```python
from build123d import *

# Parameters (mm, degrees)
SKETCH_1_R      = 2.75
EXTRUDE_1_DEPTH = 10


with BuildPart() as part:
    # Эскиз1 → Бобышка-Вытянуть1 (new body)
    # profile 1 of 2: a face of its own
    with BuildSketch(Plane.XY):
        Polygon((-16, 0), (0, 0), (0, 14), (-2, 14), (-2, 15.226497308), (-12, 21), (-16, 21), align=None)
        with Locations((-9, 8)):
            Circle(SKETCH_1_R, mode=Mode.SUBTRACT)
    # profile 2 of 2: a face of its own
    with BuildSketch(Plane.XY):
        Polygon((0, 14), (0, 0), (16, 0), (16, 21), (12, 21), (2, 15.226497308), (2, 14), align=None)
        with Locations((9, 8)):
            Circle(SKETCH_1_R, mode=Mode.SUBTRACT)
    extrude(amount=EXTRUDE_1_DEPTH)


solid = part.part
```
Verification items for the finished model (mm, model axes). A direction names the side the tool comes from. Give positions to 0.01 mm unless a question says otherwise; leave off trailing zeros. Loops run counter-clockwise (first coordinate to the right, second up) from the corner with the lowest first, then second, coordinate; pieces in that order, holes last.
1. Section check D-D, the plane y = 16. Enter the section's corners in (x, z), then the cut area to 3 significant figures.
2. Set-up check for faces 1 (the flat face through (-2, 15, 5)), 2 (the flat face through (-14, 21, 5)): record each of +Z, -Z, +X, -X, +Y, -Y from which the full face is reachable in a straight line by a thin tool's end or side.
3. Go/stop test with flat-tipped pins: pin 1 Ø12 at (x, y) = (9, 16) entering from -Z; pin 2 Ø2 at (x, z) = (-0.5, 5) entering from +Y; pin 3 Ø1 at (x, y) = (-4, 18.5) entering from -Z. Record where each tip stops, or that it passes through.
4. Section check C-C, the plane z = 7. Enter the section's corners in (x, y).
5. Section check A-A, the plane y = 8. Enter the section's corners in (x, z).
6. Mould release check, pull along X, two halves, no side actions. Record for faces 3 (the flat face through (7.07, 18.154, 4.93)), 4 (the flat face through (16, 10, 5)), 5 (the flat face through (0, 0, 5)): released by +X, released by -X, zero draft, split by the parting line, or undercut.
7. Section check B-B, the plane x = -9. Enter the section's corners in (y, z).
8. Thickness scan on line 1 (X direction, y = 6.5, z = 4.5); line 2 (X direction, y = 14.75, z = 4.25); line 3 (Y direction, x = 1.5, z = 9.5). Record the ranges inside material, lowest first.
Geometry says:
1. outline: (-16, 0) - (-3.34, 0) - (-3.34, 10) - (-16, 10) - close; (3.34, 0) - (16, 0) - (16, 10) - (3.34, 10) - close
1. area: 253 mm2
2. face 1: +Z, -Z, +Y
2. face 2: +Z, -Z, +X, -X, +Y
3. pin 1: stops at z = 0
3. pin 2: stops at y = 14
3. pin 3: passes through
4. outline: (-16, 0) - (16, 0) - (16, 21) - (12, 21) - (2, 15.23) - (2, 14) - (-2, 14) - (-2, 15.23) - (-12, 21) - (-16, 21) - close; hole circle Ø5.5 at (-9, 8); hole circle Ø5.5 at (9, 8)
5. outline: (-16, 0) - (-11.75, 0) - (-11.75, 10) - (-16, 10) - close; (-6.25, 0) - (6.25, 0) - (6.25, 10) - (-6.25, 10) - close; (11.75, 0) - (16, 0) - (16, 10) - (11.75, 10) - close
6. face 3: undercut
6. face 4: released by +X
6. face 5: zero draft
7. outline: (0, 0) - (5.25, 0) - (5.25, 10) - (0, 10) - close; (10.75, 0) - (19.27, 0) - (19.27, 10) - (10.75, 10) - close
8. line 1: x = -16 to -11.3, -6.7 to 6.7, 11.3 to 16
8. line 2: x = -16 to -2, 2 to 16
8. line 3: y = 0 to 14
